from build123d import *

# Parameters (mm, degrees)
FILLET1_R     = 3
CHAMFER1_SIZE = 1
FILLET2_R     = 1


with BuildPart() as part:
    # Sketch1 → Revolve1 (revolve)
    with BuildSketch(Plane.XY, mode=Mode.PRIVATE) as revolve1_sk:
        Polygon((6, 10.999045222), (2.5, 10.999045222), (2.5, 3.5), (0, 3.5), (0, 0), (5.062177826, 0), (13.75, -5.015916471), (15.887822174, -5.015916471), (15.887822174, -1.515916471), (14.687822174, -1.515916471), (6, 3.5), align=None)
    revolve(revolve1_sk.sketch.rotate(Axis((0, 31.975823544, 0), (0, -1, 0)), 90), axis=Axis((0, 31.975823544, 0), (0, -1, 0)))

    # Fillet1
    fillet1_edges = [part.edges().sort_by_distance(p)[0] for p in [
        (0, -5.015916471, -13.75),
    ]]
    fillet(fillet1_edges, radius=FILLET1_R)

    # Chamfer1
    chamfer1_edges = [part.edges().sort_by_distance(p)[0] for p in [
        (0, 10.999045222, -6),
    ]]
    chamfer(chamfer1_edges, length=CHAMFER1_SIZE)

    # Fillet2
    fillet2_edges = [part.edges().sort_by_distance(p)[0] for p in [
        (0, -1.515916471, -14.687822174),
    ]]
    fillet(fillet2_edges, radius=FILLET2_R)

    # Sketch4 → M3 Tapped Hole1 (revolve, cut)
    with BuildSketch(Plane(origin=(-6, 7.249522611, 0), x_dir=(0, 0, 1), z_dir=(0, 1, 0))):
        Polygon((0, 0), (0, 7.251075774), (1.25, 6.5), (1.25, 0.275), (1.525, 0), align=None)
    revolve(axis=Axis((-12.35, 7.249522611, 0), (1, 0, 0)), mode=Mode.SUBTRACT)


solid = part.part
The model under review builds one solid part; all positions refer to its coordinate system, in mm. A direction names the side the tool comes from. Round coordinates to 2 decimals unless told otherwise and drop trailing zeros. Order: outer loops, then holes, each group sorted by start corner. A loop starts at its lowest first (then second) coordinate and runs counter-clockwise, first axis right, second up. Notation, with made-up numbers: (62.5, -21.5) -> (108.5, -21.5) arc R25 ccw to (108.5, -3.5) -> close; hole circle Ø10 at (88.25, -9). An arc over 180 degrees is marked (long way). Use CSV: the item, a comma, the result in double quotes. Start each with the question number.
(1) Insertion check: pin 1 (1.5 mm diameter, centred on x = -4.5, y = 6, fed in from +Z); pin 2 (6 mm diameter, centred on x = -7, y = -3, fed in from -Z); pin 3 (1 mm diameter, centred on y = 0.5, z = -0.5, fed in from +X); pin 4 (9.5 mm diameter, centred on x = 5, z = -7, fed in from +Y). Each pin has a flat end and moves straight along its axis. Give the tip position at first contact, or say it passes through.
(2) Consider section D-D on y = 1.75. Write out the cut boundary in (x, z).
(3) Consider section B-B on x = 0. Write out the cut boundary in (y, z), and give its area (3 significant figures).
(4) Wall thickness on probe 1 along Y at (x, z) = (-3.1, 0); probe 2 along X at (y, z) = (5, 0); probe 3 along Y at (x, z) = (2, -0.5): over which ranges is each line inside the solid? List them lowest first. Write a range as from..to.
(5) Mouldability with a two-part tool opening along X and no side actions: class faces 1 (the face through (0, 3.5, 0)), 2 (the face through (2, 10.999, 2)), 3 (the face through (15.51, -3.24, -3.44)) as pulls with the +X half, pulls with the -X half, needs draft (parallel to the pull), parting line crosses it, or undercut.
(6) Tool access review of faces 4 (the face through (0, 0, 0)), 5 (the face through (2.44, 7.2, -0.54)), 6 (the face through (-3.97, 7.19, -1.25)), 7 (the face through (7, -5.016, -13)): name each direction out of +Z, -Z, +X, -X, +Y, -Y from which nothing blocks a thin tool from reaching the whole face with its end or side.
(7) Consider section C-C on y = 5. Write out the cut boundary in (x, z).
Responses:
1,pin 1,"z = 4.68"
1,pin 2,"z = -15.38"
1,pin 3,"x = 12.05"
1,pin 4,"y = 11"
2,outline,"circle Ø18.06 at (0, 0)"
3,outline,"(-5.02, -15.89) -> (-1.52, -15.89) -> (-1.52, -14.96) arc R1 cw to (-1.38, -14.46) -> (3.5, -6) -> (10, -6) -> (11, -5) -> (11, -2.5) -> (3.5, -2.5) -> (3.5, 2.5) -> (11, 2.5) -> (11, 5) -> (10, 6) -> (3.5, 6) -> (-1.38, 14.46) arc R1 cw to (-1.52, 14.96) -> (-1.52, 15.89) -> (-5.02, 15.89) -> (-5.02, 14.55) arc R3 ccw to (-4.61, 13.05) -> (0, 5.06) -> (0, -5.06) -> (-4.61, -13.05) arc R3 ccw to (-5.02, -14.55) -> close"
3,area,"172 mm²"
4,probe 1,"0..6, 8.5..11"
4,probe 2,"-6..-2.5, 2.5..6"
4,probe 3,"0..3.5"
5,face 1,"undercut"
5,face 2,"needs draft"
5,face 3,"parting line crosses it"
6,face 4,"-Y"
6,face 5,"+Y"
6,face 6,"-X"
6,face 7,"+Z, -Z, +X, -X, -Y"
7,outline,"circle Ø12 at (0, 0); hole circle Ø5 at (0, 0)"
